Build history of the part. All positions in model axes, mm. A direction names the side the tool comes from. Round coordinates to 2 decimals unless told otherwise and drop trailing zeros. Loops run counter-clockwise (first coordinate to the right, second up) from the corner with the lowest first, then second, coordinate; pieces in that order, holes last. Notation, with made-up numbers: M 48,64 L 54,64 A15 ccw 54,82 Z; hole C -6.75,84 d5. An arc over 180 degrees is marked long. One line per item, written item: value.
```python
from build123d import *

# Parameters (mm, degrees)
SKETCH1_W           = 80
SKETCH1_H           = 80
BOSS_EXTRUDE1_DEPTH = 20
SKETCH3_R           = 4.5
CUT_EXTRUDE2_DEPTH  = 92.651513899
SKETCH3_4_R         = 7.65
SKETCH3_4_R_2       = 4.5
CUT_EXTRUDE3_DEPTH  = 24.5
SKETCH7_R           = 4.5
CUT_EXTRUDE4_DEPTH  = 92.651513899
SKETCH7_4_R         = 7.65
SKETCH7_4_R_2       = 4.5
CUT_EXTRUDE5_DEPTH  = 24.5
FILLET1_R           = 1
SKETCH8_R           = 2.55
CUT_EXTRUDE7_DEPTH  = 70.282032303


with BuildPart() as part:
    # Sketch1 → Boss-Extrude1 (new, symmetric)
    with BuildSketch(Plane(origin=(0, 0, 0), x_dir=(1, 0, 0), z_dir=(0, 1, 0))):
        Rectangle(SKETCH1_W, SKETCH1_H)
    extrude(amount=BOSS_EXTRUDE1_DEPTH, both=True)

    # Sketch3 → Cut-Extrude2 (cut, through all)
    with BuildSketch(Plane.XY.offset(40)):
        with Locations((-30, -10.5)):
            Circle(SKETCH3_R)
        with Locations(Location((30, -10.5, 0), (0, 0, 180))):
            Circle(SKETCH3_R)
    extrude(amount=-CUT_EXTRUDE2_DEPTH, mode=Mode.SUBTRACT)

    # Sketch3_4 → Cut-Extrude3 (cut)
    # profile 1 of 2: a face of its own
    with BuildSketch(Plane.XY.offset(40)):
        with Locations((-30, -10.5)):
            Circle(SKETCH3_4_R)
        with Locations((-30, -10.5)):
            Circle(SKETCH3_4_R_2, mode=Mode.SUBTRACT)
    # profile 2 of 2: a face of its own
    with BuildSketch(Plane.XY.offset(40)):
        with Locations(Location((30, -10.5, 0), (0, 0, 180))):
            Circle(SKETCH3_4_R)
        with Locations(Location((30, -10.5, 0), (0, 0, 180))):
            Circle(SKETCH3_4_R_2, mode=Mode.SUBTRACT)
    cut_extrude3 = extrude(amount=-CUT_EXTRUDE3_DEPTH, mode=Mode.SUBTRACT)

    # Mirror1: Cut-Extrude3 across plane
    add(cut_extrude3.mirror(Plane.XY), mode=Mode.SUBTRACT)

    # Sketch7 → Cut-Extrude4 (cut, through all)
    with BuildSketch(Plane(origin=(40, 0, 0), x_dir=(0, 0, -1), z_dir=(1, 0, 0))):
        with Locations((-30, 10.5)):
            Circle(SKETCH7_R)
        with Locations(Location((30, 10.5, 0), (0, 0, 180))):
            Circle(SKETCH7_R)
    extrude(amount=-CUT_EXTRUDE4_DEPTH, mode=Mode.SUBTRACT)

    # Sketch7_4 → Cut-Extrude5 (cut)
    # profile 1 of 2: a face of its own
    with BuildSketch(Plane(origin=(40, 0, 0), x_dir=(0, 0, -1), z_dir=(1, 0, 0))):
        with Locations((-30, 10.5)):
            Circle(SKETCH7_4_R)
        with Locations((-30, 10.5)):
            Circle(SKETCH7_4_R_2, mode=Mode.SUBTRACT)
    # profile 2 of 2: a face of its own
    with BuildSketch(Plane(origin=(40, 0, 0), x_dir=(0, 0, -1), z_dir=(1, 0, 0))):
        with Locations(Location((30, 10.5, 0), (0, 0, 180))):
            Circle(SKETCH7_4_R)
        with Locations(Location((30, 10.5, 0), (0, 0, 180))):
            Circle(SKETCH7_4_R_2, mode=Mode.SUBTRACT)
    cut_extrude5 = extrude(amount=-CUT_EXTRUDE5_DEPTH, mode=Mode.SUBTRACT)

    # Mirror2: Cut-Extrude5 across plane
    add(cut_extrude5.mirror(Plane(origin=(0, 0, 0), x_dir=(0, 0, 1), z_dir=(1, 0, 0))), mode=Mode.SUBTRACT)

    # Fillet1
    fillet1_edges = [part.edges().sort_by_distance(p)[0] for p in [
        (40, 20, 0),
        (0, 20, -40),
        (-40, 20, 0),
        (0, -20, -40),
        (40, -20, 0),
        (0, -20, 40),
        (-40, -20, 0),
        (-40, 0, -40),
        (40, 0, -40),
        (40, 0, 40),
        (-40, 0, 40),
        (0, 20, 40),
    ]]
    fillet(fillet1_edges, radius=FILLET1_R)

    # Sketch8 → Cut-Extrude7 (cut, through all)
    with BuildSketch(Plane(origin=(0, 20, 0), x_dir=(1, 0, 0), z_dir=(0, 1, 0))):
        with Locations(Location((-17.5, 15, 0), (0, 0, 270))):
            Circle(SKETCH8_R)
        with Locations(Location((12.5, 15, 0), (0, 0, 270))):
            Circle(SKETCH8_R)
        with Locations(Location((12.5, -15, 0), (0, 0, 270))):
            Circle(SKETCH8_R)
        with Locations(Location((-17.5, -15, 0), (0, 0, 270))):
            Circle(SKETCH8_R)
    extrude(amount=-CUT_EXTRUDE7_DEPTH, mode=Mode.SUBTRACT)


solid = part.part
```
Item 1: Drop flat-ended pins along their axis: P1, Ø11.5, axis at x = -30, y = -10.5, coming from the -Z side; P2, Ø14.5, axis at x = 30, y = -10.5, coming from the +Z side; P3, Ø12, axis at y = 10.5, z = 30, coming from the +X side. Give the stop position or say it passes through.
Check values:
P1: stops at z = -15.5
P2: stops at z = 15.5
P3: stops at x = 15.5
Item 2: Which spindle directions (+Z, -Z, +X, -X, +Y, -Y) get a long thin tool onto all of the face, cutting with end or side? Do faces 4 (the face through (35.64, -15.67, 27.92)), 5 (the face through (-15.5, 7.2, 26.7)), 6 (the face through (27.922, 10.164, -37.643)). Say none if no direction does.
Check values:
face 4: +Z
face 5: -X
face 6: +X
Item 3: Pull direction Z, two halves, no side cores. Call faces 1 (the face through (-36.071, -15.155, -27.922)), 2 (the face through (15.5, 7.2, 26.7)), 3 (the face through (-1, 0, 40)): pulls with the +Z half, pulls with the -Z half, needs draft (parallel to the pull), parting line crosses it, or undercut.
Check values:
face 1: needs draft
face 2: undercut
face 3: pulls with the +Z half
Item 4: Slice it at A-A, the plane x = -30. Give the cut face in (y, z), and give its area (3 significant figures).
Check values:
outline: M -20,-39 A1 ccw -19,-40 L -18.15,-40 L -18.15,-15.5 L -15,-15.5 L -15,15.5 L -18.15,15.5 L -18.15,40 L -19,40 A1 ccw -20,39 Z; M -6,-15.5 L -2.85,-15.5 L -2.85,-40 L 19,-40 A1 ccw 20,-39 L 20,39 A1 ccw 19,40 L -2.85,40 L -2.85,15.5 L -6,15.5 Z; hole C 10.5,-30 d15.3; hole C 10.5,30 d15.3
area: 1,800 mm2
Item 5: Slice it at C-C, the plane x = -17.5. Give the cut face in (y, z).
Check values:
outline: M -20,-39 A1 ccw -19,-40 L 19,-40 A1 ccw 20,-39 L 20,-17.55 L -20,-17.55 Z; M -20,-12.45 L 20,-12.45 L 20,12.45 L -20,12.45 Z; M -20,17.55 L 20,17.55 L 20,39 A1 ccw 19,40 L -19,40 A1 ccw -20,39 Z; hole C 10.5,-30 d15.3; hole C 10.5,30 d15.3
Item 6: Slice it at B-B, the plane z = -30. Give the cut face in (x, y).
Check values:
outline: M -40,-19 A1 ccw -39,-20 L 39,-20 A1 ccw 40,-19 L 40,2.85 L 15.5,2.85 L 15.5,6 L -15.5,6 L -15.5,2.85 L -40,2.85 Z; M -40,18.15 L -15.5,18.15 L -15.5,15 L 15.5,15 L 15.5,18.15 L 40,18.15 L 40,19 A1 ccw 39,20 L -39,20 A1 ccw -40,19 Z; hole C -30,-10.5 d15.3; hole C 30,-10.5 d15.3
Item 7: Wall check: line 1 along X through (y, z) = (-10, 25); line 2 along Z through (x, y) = (37.5, 15); line 3 along Y through (x, z) = (21.5, 30). Give the ranges that are in metal, low to high.
Check values:
line 1: x = -40 to -37.63, -22.37 to 22.37, 37.63 to 40
line 2: z = -40 to -36.19, -23.81 to 23.81, 36.19 to 40
line 3: y = -20 to 2.85, 18.15 to 20
Item 8: Slice it at D-D, the plane y = 10.5. Give the number of separate pieces and of enclosed holes in the cut face, and give its area (3 significant figures).
Check values:
separate pieces: 3
enclosed holes: 4
area: 4,260 mm2
